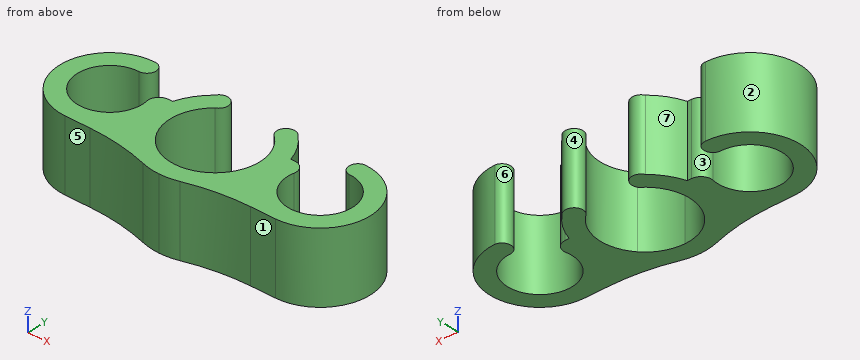
```python
from build123d import *

# Parameters (mm, degrees)
F1_DEPTH = 12
F2_R     = 35.487136
F3_R     = 1.788944


with BuildPart() as f1:
    # F0 (on Top) → F1 (new body)
    with BuildSketch(Plane.XY):
        with BuildLine():
            Line((0, -7.6), (0, -10.6))
            ThreePointArc((0, -10.6), (3.336165, -10.061312), (6.333246, -8.5))
            Line((6.333246, -8.5), (18, -8.5))
            ThreePointArc((18, -8.5), (26.5, 0), (18, 8.5))
            Line((18, 8.5), (18, 5.5))
            ThreePointArc((18, 5.5), (20.530042, -4.883532), (13.507076, 3.172323))
            Line((13.507076, 3.172323), (10.114167, 3.172323))
            ThreePointArc((10.114167, 3.172323), (8.93073, 5.709821), (7.124192, 7.848942))
            ThreePointArc((7.124192, 7.848942), (4.718849, 8.006432), (5.107912, 5.627543))
            ThreePointArc((5.107912, 5.627543), (7.586173, 0.45824), (5.748161, -4.971785))
            ThreePointArc((5.748161, -4.971785), (3.160256, -6.911786), (0, -7.6))
        make_face()
        with BuildLine():
            Line((18, 5.5), (18, 8.5))
            ThreePointArc((18, 8.5), (16.655563, 7), (18, 5.5))
        make_face()
        with BuildLine():
            ThreePointArc((-6.333246, -8.5), (-3.336165, -10.061312), (0, -10.6))
            Line((0, -10.6), (0, -7.6))
            ThreePointArc((0, -7.6), (-7.089758, -2.737761), (-5.107912, 5.627543))
            ThreePointArc((-5.107912, 5.627543), (-4.563236, 8.147676), (-7.124192, 7.848942))
            ThreePointArc((-7.124192, 7.848942), (-8.93073, 5.709821), (-10.114167, 3.172323))
            Line((-10.114167, 3.172323), (-13.507076, 3.172323))
            ThreePointArc((-13.507076, 3.172323), (-20.530042, -4.883532), (-18, 5.5))
            Line((-18, 5.5), (-18, 8.5))
            ThreePointArc((-18, 8.5), (-26.5, 0), (-18, -8.5))
            Line((-18, -8.5), (-6.333246, -8.5))
        make_face()
        with BuildLine():
            ThreePointArc((-18, 5.5), (-16.428817, 7), (-18, 8.5))
            Line((-18, 8.5), (-18, 5.5))
        make_face()
    extrude(amount=F1_DEPTH)

    # F2
    f2_edges = [f1.edges().sort_by_distance(p)[0] for p in [
        (-6.333246, -8.5, 6),
        (6.333246, -8.5, 6),
    ]]
    fillet(f2_edges, radius=F2_R)

    # F3
    f3_edges = [f1.edges().sort_by_distance(p)[0] for p in [
        (-13.507076, 3.172323, 6),
        (13.507076, 3.172323, 6),
    ]]
    fillet(f3_edges, radius=F3_R)


solid = f1.part
```
Verification items for the finished model (mm, model axes). Face numbers are marked on the shaded views. A direction names the side the tool comes from. Round coordinates to 2 decimals unless told otherwise and drop trailing zeros. Write each loop counter-clockwise with the first axis right and the second up, starting at its lowest first coordinate (ties: lowest second). Pieces come first, ordered by that corner, then holes. Notation, with made-up numbers: (-11.5, 52.5) - (28.5, 52.5) arc R21 cw to (28.5, 64.5) - close; hole circle Ø3 at (43, 46). An arc over 180 degrees is marked (long way). Answer as a JSON object with one key per item and string values. Group by question number.
Q1. Mould release check, pull along X, two halves, no side actions. Record for the marked faces 1, 2, 3 and 4: released by +X, released by -X, zero draft, split by the parting line, or undercut.
Q2. Section check C-C, the plane y = -3. Enter the section's corners in (x, z).
Q3. Section check D-D, the plane z = 4.75. Enter the section's corners in (x, y) (3 decimals).
Q4. Thickness scan on line 1 (Y direction, x = -18, z = 5.25); line 2 (X direction, y = -0.75, z = 3.75); line 3 (X direction, y = -1.25, z = 1.75). Record the ranges inside material, lowest first.
Q5. Tool access check on the marked faces 5, 6 and 7. Record the directions out of +Z, -Z, +X, -X, +Y, -Y that give a thin tool (end or side, any length) a straight path to the whole face; none if there is none.
Q6. Section check B-B, the plane y = 0. Enter the section's corners in (x, z).
Q7. Section check A-A, the plane x = 6.5. Enter the section's corners in (y, z).
Q8. Go/stop test with flat-tipped pins: pin 1 Ø5 at (x, y) = (3, -3.5) entering from +Z; pin 2 Ø4.5 at (x, z) = (17, 8) entering from -Y; pin 3 Ø3 at (x, z) = (-20.5, 7.5) entering from +Y; pin 4 Ø6 at (x, z) = (11, 8) entering from -Y. Record where each tip stops, or that it passes through.
Found:
{
 "1": {"face 1": "zero draft", "face 2": "released by -X", "face 3": "undercut", "face 4": "undercut"},
 "2": {"outline": "(-25.95, 0) - (-22.61, 0) - (-22.61, 12) - (-25.95, 12) - close; (-13.39, 0) - (-6.98, 0) - (-6.98, 12) - (-13.39, 12) - close; (6.98, 0) - (13.39, 0) - (13.39, 12) - (6.98, 12) - close; (22.61, 0) - (25.95, 0) - (25.95, 12) - (22.61, 12) - close"},
 "3": {"outline": "(-18, -8.5) - (-13.753, -8.5) arc R35.487 cw to (-3.163, -10.117) arc R10.6 ccw to (0, -10.6) arc R10.6 ccw to (3.163, -10.117) arc R35.487 cw to (13.753, -8.5) - (18, -8.5) arc R8.5 ccw to (18, 8.5) arc R1.509 ccw to (18, 5.5) arc R5.5 cw (long way) to (12.6, 1.044) arc R1.789 ccw to (10.844, 3.172) - (10.114, 3.172) arc R10.6 ccw to (7.124, 7.849) arc R1.54 ccw (long way) to (5.108, 5.628) arc R7.6 cw to (5.748, -4.972) arc R7.6 cw to (0, -7.6) arc R7.6 cw to (-5.108, 5.628) arc R1.585 ccw (long way) to (-7.124, 7.849) arc R10.6 ccw to (-10.114, 3.172) - (-10.844, 3.172) arc R1.789 ccw to (-12.6, 1.044) arc R5.5 cw (long way) to (-18, 5.5) arc R1.502 ccw (long way) to (-18, 8.5) arc R8.5 ccw to start"},
 "4": {"line 1": "y = -8.5 to -5.5, 5.5 to 8.5", "line 2": "x = -26.47 to -23.45, -12.55 to -7.56, 7.56 to 12.55, 23.45 to 26.47", "line 3": "x = -26.41 to -23.36, -12.64 to -7.5, 7.5 to 12.64, 23.36 to 26.41"},
 "5": {"face 5": "+Z, -Z, -X, -Y", "face 6": "+Z, -Z", "face 7": "+Z, -Z, +Y"},
 "6": {"outline": "(-26.5, 0) - (-23.5, 0) - (-23.5, 12) - (-26.5, 12) - close; (-12.5, 0) - (-7.6, 0) - (-7.6, 12) - (-12.5, 12) - close; (7.6, 0) - (12.5, 0) - (12.5, 12) - (7.6, 12) - close; (23.5, 0) - (26.5, 0) - (26.5, 12) - (23.5, 12) - close"},
 "7": {"outline": "(-9.25, 0) - (-3.94, 0) - (-3.94, 12) - (-9.25, 12) - close; (3.94, 0) - (8.37, 0) - (8.37, 12) - (3.94, 12) - close"},
 "8": {"pin 1": "passes through", "pin 2": "stops at y = -8.5", "pin 3": "stops at y = 8.44", "pin 4": "stops at y = -8.97"}
}
